```python
from build123d import *

# Parameters (mm, degrees)
SKETCH2_W           = 177.8
SKETCH2_H           = 31.75
BASE_BLUE_DEPTH     = 76.2
BASE_YELLOW_R_DEPTH = 12.7
BASE_YELLOW_L_DEPTH = 12.7
SKETCH3_R           = 6.5532
CYL_RED_DEPTH       = 32.75


with BuildPart() as part:
    # Sketch2 → base-blue (new body)
    with BuildSketch(Plane.XY):
        Rectangle(SKETCH2_W, SKETCH2_H)
    extrude(amount=-BASE_BLUE_DEPTH)

    # Sketch4 → base-yellow-R (add)
    with BuildSketch(Plane.XY):
        with BuildLine():
            Line((44.45, 15.875), (-44.45, 15.875))
            ThreePointArc((-44.45, 15.875), (-66.900640303, 6.575640303), (-76.2, -15.875))
            Line((-76.2, -15.875), (-63.5, -15.875))
            ThreePointArc((-63.5, -15.875), (-44.45, 3.175), (-25.4, -15.875))
            Line((-25.4, -15.875), (25.4, -15.875))
            ThreePointArc((25.4, -15.875), (44.45, 3.175), (63.5, -15.875))
            Line((63.5, -15.875), (76.2, -15.875))
            ThreePointArc((76.2, -15.875), (66.900640303, 6.575640303), (44.45, 15.875))
        make_face()
    extrude(amount=BASE_YELLOW_R_DEPTH)

    # Sketch5 → base-yellow-L (add)
    with BuildSketch(Plane(origin=(0, 0, -76.2), x_dir=(-1, 0, 0), z_dir=(0, 0, -1))):
        with BuildLine():
            Line((76.2, -15.875), (63.5, -15.875))
            ThreePointArc((63.5, -15.875), (44.45, 3.175), (25.4, -15.875))
            Line((25.4, -15.875), (-25.4, -15.875))
            ThreePointArc((-25.4, -15.875), (-44.45, 3.175), (-63.5, -15.875))
            Line((-63.5, -15.875), (-76.2, -15.875))
            ThreePointArc((-76.2, -15.875), (-66.900640303, 6.575640303), (-44.45, 15.875))
            Line((-44.45, 15.875), (44.45, 15.875))
            ThreePointArc((44.45, 15.875), (66.900640303, 6.575640303), (76.2, -15.875))
        make_face()
    extrude(amount=BASE_YELLOW_L_DEPTH)

    # Sketch3 → cyl-red (cut, through all)
    with BuildSketch(Plane(origin=(0, 15.875, 0), x_dir=(1, 0, 0), z_dir=(0, 1, 0))):
        with Locations((-76.2, 19.05)):
            Circle(SKETCH3_R)
        with Locations((-76.2, 57.15)):
            Circle(SKETCH3_R)
        with Locations((76.2, 57.15)):
            Circle(SKETCH3_R)
        with Locations((76.2, 19.05)):
            Circle(SKETCH3_R)
        Circle(SKETCH3_R)
        with Locations((0, 76.2)):
            Circle(SKETCH3_R)
    extrude(amount=-CYL_RED_DEPTH, mode=Mode.SUBTRACT)


solid = part.part
```
Geometry check sheet. Reference: the model listing, model coordinates, mm. A direction names the side the tool comes from. Coordinates: 2 decimals unless noted, no trailing zeros. Loops run counter-clockwise (first coordinate to the right, second up) from the corner with the lowest first, then second, coordinate; pieces in that order, holes last. Notation, with made-up numbers: (-37, 53) - (-1, 53) arc R22 cw to (-1, 62) - close; hole circle Ø3 at (17.25, -13). An arc over 180 degrees is marked (long way). One line per item, written item: value. Start each with the question number.
(1) Cross-section at D-D on z = -3. Enter the section's corners in (x, y) (3 decimals), plus the area to 3 significant figures.
(2) Material ranges on line 1 (X direction, y = 0, z = -19.05); line 2 (Z direction, x = -76.2, y = 4); line 3 (Z direction, x = -71, y = -10), recorded low to high. Write a range as [from, to].
(3) Cross-section at B-B on z = -57.15. Enter the section's corners in (x, y) (3 decimals).
(4) Cross-section at A-A on x = 0. Enter the section's corners in (y, z) (3 decimals).
(5) Cross-section at C-C on y = -1. Count the separate pieces of the cut face and the enclosed holes in it, plus the area to 3 significant figures.
(6) Mould release check, pull along X, two halves, no side actions. Record for faces 1 (the flat face through (76, 4, -76.2)), 2 (the cylindrical face through (-66.652, 6.821, 6.261)), 3 (the flat face through (-45, -8, 0)): released by +X, released by -X, zero draft, split by the parting line, or undercut.
(7) Depth check by flat-ended pin: P1, Ø5.5, axis at x = -51.5, y = -5.5, coming from the +Z side; P2, Ø5.5, axis at x = 45, y = -6, coming from the -Z side. Enter the tip coordinate at first touch or a pass-through.
(8) Tool access check on faces 4 (the flat face through (44, -8, -76.2)), 5 (the flat face through (-77, 4, 0)), 6 (the flat face through (44, -8, 0)), 7 (the cylindrical face through (67.146, 6.327, 6.261)), 8 (the flat face through (-77, 4, -76.2)). Record the directions out of +Z, -Z, +X, -X, +Y, -Y that give a thin tool (end or side, any length) a straight path to the whole face; none if there is none.
Results below:
1. outline: (-88.9, -15.875) - (-5.826, -15.875) - (-5.826, 15.875) - (-88.9, 15.875) - close; (5.826, -15.875) - (88.9, -15.875) - (88.9, 15.875) - (5.826, 15.875) - close
1. area: 5,280 mm2
2. line 1: x = [-88.9, -82.75], [-69.65, 69.65], [82.75, 88.9]
2. line 2: z = [-76.2, -63.7], [-50.6, -25.6], [-12.5, 0]
2. line 3: z = [-88.9, -61.14], [-53.16, -23.04], [-15.06, 12.7]
3. outline: (-88.9, -15.875) - (-82.753, -15.875) - (-82.753, 15.875) - (-88.9, 15.875) - close; (-69.647, -15.875) - (69.647, -15.875) - (69.647, 15.875) - (-69.647, 15.875) - close; (82.753, -15.875) - (88.9, -15.875) - (88.9, 15.875) - (82.753, 15.875) - close
4. outline: (-15.875, -88.9) - (15.875, -88.9) - (15.875, -82.753) - (-15.875, -82.753) - close; (-15.875, -69.647) - (15.875, -69.647) - (15.875, -6.553) - (-15.875, -6.553) - close; (-15.875, 6.553) - (15.875, 6.553) - (15.875, 12.7) - (-15.875, 12.7) - close
5. separate pieces: 1
5. enclosed holes: 6
5. area: 15,200 mm2
6. face 1: zero draft
6. face 2: released by -X
6. face 3: undercut
7. P1: stops at z = 0
7. P2: stops at z = -76.2
8. face 4: -Z, -Y
8. face 5: +Z, -X, +Y
8. face 6: +Z, -Y
8. face 7: +Z, +X, +Y
8. face 8: -Z, -X, +Y
